For this review, take the finished solid that the model builds, in its own axes (mm). A direction names the side the tool comes from. Round coordinates to 2 decimals unless told otherwise and drop trailing zeros. Order: outer loops, then holes, each group sorted by start corner. A loop starts at its lowest first (then second) coordinate and runs counter-clockwise, first axis right, second up. Notation, with made-up numbers: (48, 70) - (62, 70) arc R19 cw to (62, 95) - close; hole circle Ø11 at (27.5, 33). An arc over 180 degrees is marked (long way). One line per item, written item: value.
```python
from build123d import *

# Parameters (mm, degrees)
SKETCH_R        = 13
SKETCH_R_2      = 8.1
PAD_DEPTH       = 10
SKETCH001_R     = 13
SKETCH001_R_2   = 7
PAD001_DEPTH    = 20
CHAMFER_SIZE    = 0.4
CHAMFER001_SIZE = 0.4


with BuildPart() as part:
    # Sketch → Pad (new body)
    with BuildSketch(Plane.XY):
        Circle(SKETCH_R)
        Circle(SKETCH_R_2, mode=Mode.SUBTRACT)
    extrude(amount=PAD_DEPTH)

    # Sketch001 (on Face4 of Pad) → Pad001 (join)
    with BuildSketch(Plane.XY.offset(10)):
        Circle(SKETCH001_R)
        Circle(SKETCH001_R_2, mode=Mode.SUBTRACT)
    extrude(amount=PAD001_DEPTH)

    # Chamfer
    chamfer_edges = [part.edges().sort_by_distance(p)[0] for p in [
        (-8.1, 0, 0),
    ]]
    chamfer(chamfer_edges, length=CHAMFER_SIZE)

    # Chamfer001
    chamfer001_edges = [part.edges().sort_by_distance(p)[0] for p in [
        (-13, 0, 0),
    ]]
    chamfer(chamfer001_edges, length=CHAMFER001_SIZE)


solid = part.part
```
Item 1: Wall thickness on line 1 (Y direction, x = 0, z = 25.75); line 2 (Y direction, x = 0, z = 5.5); line 3 (X direction, y = 1.25, z = 23.25): over which ranges is each line inside the solid? List them lowest first.
Returned:
line 1: -13 to -7, 7 to 13
line 2: -13 to -8.1, 8.1 to 13
line 3: -12.94 to -6.89, 6.89 to 12.94
Item 2: For P1, Ø4, axis at x = 3.5, z = 14, coming from the -Y side; P2, Ø1.5, axis at x = -7.5, z = 12.5, coming from the +Y side; P3, Ø12, axis at y = 10, z = 23.5, coming from the -X side, all flat-tipped, find the tip position at first contact; note any pin that passes through.
Returned:
P1: y = -12.91
P2: y = 11.11
P3: x = -12.37
Item 3: Machinability: for faces 1 (the flat face through (-6, -4, 10)), 2 (the flat face through (-3, -8.2, 0)), which of the approach directions +Z, -Z, +X, -X, +Y, -Y give a long, thin tool a straight path to every point of the face, cutting with its end or side? Answer none if there is none.
Returned:
face 1: -Z
face 2: -Z, +X, -X, +Y, -Y
Item 4: Take a section at D-D (z = 5.25). Write out the cut boundary in (x, y).
Returned:
outline: circle Ø26 at (0, 0); hole circle Ø16.2 at (0, 0)
Item 5: The part is to be moulded in two halves that separate along Y. For faces 3 (the cylindrical face through (6.466, -2.681, 19.86)), 4 (the flat face through (6, -6, 30)), 5 (the cylindrical face through (-10.316, -7.91, 14.993)), say which applies: +Y half, -Y half, draft (parallel to the pull), parting line (faces both ways), or undercut.
Returned:
face 3: undercut
face 4: draft
face 5: parting line
Item 6: Take a section at C-C (z = 11.5). Write out the cut boundary in (x, y).
Returned:
outline: circle Ø26 at (0, 0); hole circle Ø14 at (0, 0)
Item 7: Take a section at A-A (y = 0). Write out the cut boundary in (x, z).
Returned:
outline: (-13, 0.4) - (-12.6, 0) - (-8.5, 0) - (-8.1, 0.4) - (-8.1, 10) - (-7, 10) - (-7, 30) - (-13, 30) - close; (7, 10) - (8.1, 10) - (8.1, 0.4) - (8.5, 0) - (12.6, 0) - (13, 0.4) - (13, 30) - (7, 30) - close
